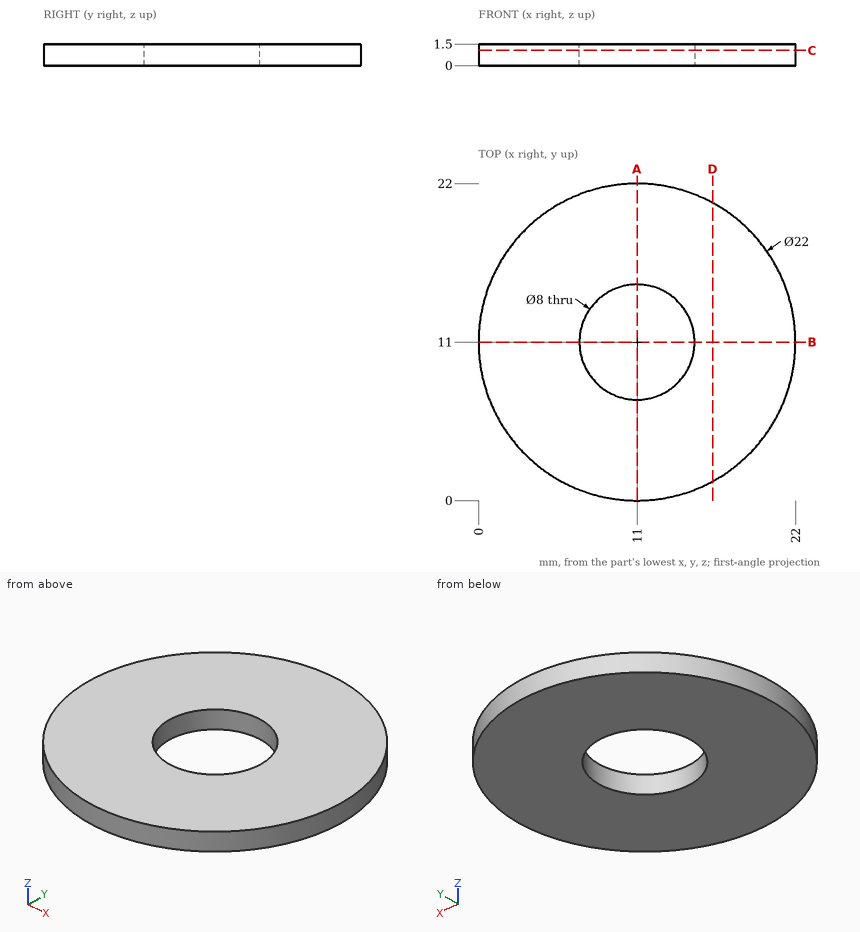
Design review of the part shown in the three views and the two pictorial views. Dimensions are in mm from the part's minimum x, y and z. Give positions to 0.01 mm unless a question says otherwise; leave off trailing zeros. Write each loop counter-clockwise with the first axis right and the second up, starting at its lowest first coordinate (ties: lowest second). Pieces come first, ordered by that corner, then holes.
(1) Add section A-A (x = 11). Give the boundary of the cut face in (y, z).
Checked values:
outline: (0, 0) - (7, 0) - (7, 1.5) - (0, 1.5) - close; (15, 0) - (22, 0) - (22, 1.5) - (15, 1.5) - close
(2) Add section C-C (z = 1.05). Give the boundary of the cut face in (x, y), and give its area (3 significant figures).
Checked values:
outline: circle Ø22 at (11, 11); hole circle Ø8 at (11, 11)
area: 330 mm2
(3) Add section D-D (x = 16.25). Give the boundary of the cut face in (y, z).
Checked values:
outline: (1.33, 0) - (20.67, 0) - (20.67, 1.5) - (1.33, 1.5) - close
(4) Wall thickness on line 1 along Y through (x, z) = (11, 0.3); line 2 along X through (y, z) = (12.5, 1.3); line 3 along Y through (x, z) = (12, 0.3): over which ranges is each line inside the solid? List them lowest first.
Checked values:
line 1: y = 0 to 7, 15 to 22
line 2: x = 0.1 to 7.29, 14.71 to 21.9
line 3: y = 0.05 to 7.13, 14.87 to 21.95
